Geometry check sheet. Reference: the model listing, model coordinates, mm. A direction names the side the tool comes from. Give positions to 0.01 mm unless a question says otherwise; leave off trailing zeros. Loops run counter-clockwise (first coordinate to the right, second up) from the corner with the lowest first, then second, coordinate; pieces in that order, holes last. Notation, with made-up numbers: (-17, 16.25) -> (2, 16.25) arc R4 ccw to (2, 20.25) -> close; hole circle Ø8 at (0.5, 35.25). An arc over 180 degrees is marked (long way). One line per item, written item: value. Start each with the question number.
(1) Sectioned sample at C-C, the plane y = 5.75. Record the cut outline in (x, z), then the cut area to 3 significant figures.
(2) Sectioned sample at D-D, the plane z = 0. State how many separate pieces and enclosed holes the cut face has, then the cut area to 3 significant figures.
(3) Gauge pin test, flat ends, axial feed: pin 1 Ø0.9 at (x, y) = (-4.5, -4) entering from +Z; pin 2 Ø1 at (y, z) = (-4.5, 0) entering from -X; pin 3 Ø4 at (x, z) = (-7.5, 2) entering from -Y (3 decimals). Record the tip position at first contact, or that the pin passes through.
(4) Sectioned sample at A-A, the plane x = -1.75. Record the cut outline in (y, z) (3 decimals), then the cut area to 3 significant figures.
(5) Draft check along Z on faces 1 (the face through (-4.544, -6.675, -0.011)), 2 (the face through (4.25, -5.3, -0.7)), 3 (the face through (0, 0, -3.4)). Enter one of: pulls with the +Z half, pulls with the -Z half, needs draft (parallel to the pull), parting line crosses it, or undercut.
(6) Tool access check on faces 4 (the face through (-4.544, -4.675, 0.011)), 5 (the face through (-7, 3.025, 0)), 6 (the face through (-0.35, -5.3, -0.7)), 7 (the face through (3.1, 6, 0)). Record the directions out of +Z, -Z, +X, -X, +Y, -Y that give a thin tool (end or side, any length) a straight path to the whole face; none if there is none.
(7) Sectioned sample at B-B, the plane z = -2.5. Record the cut outline in (x, y) (3 decimals), then the cut area to 3 significant figures.
(8) Scan lines: line 1 along X through (y, z) = (-4, -0.5); line 2 along Y through (x, z) = (5, 0) (3 decimals). Record each from-to range of solid material in increasing order. Write a range as from..to.
from build123d import *

# Parameters (mm, degrees)
BOSS_EXTRU_1_DEPTH      = 3.4
BOSS_EXTRU_1_DEPTH_BACK = 3.4
ENL_V_MAT_EXTRU_1_DEPTH = 6.8
ESQUISSE4_W             = 6.2
ESQUISSE4_H             = 4.2
ENL_V_MAT_EXTRU_2_DEPTH = 0.3
BOSS_EXTRU_2_DEPTH      = 1.95
BOSS_EXTRU_2_DEPTH_BACK = 1.95
ESQUISSE7_W             = 0.8
ESQUISSE7_H             = 2
BOSS_EXTRU_3_DEPTH      = 4.2
CONG_1_R                = 0.5
ENL_V_MAT_EXTRU_3_DEPTH = 10.2


with BuildPart() as part:
    # Esquisse1 → Boss.-Extru.1 (new body, two sides)
    with BuildSketch(Plane.XY) as boss_extru_1_sk:
        Polygon((-6.45, 3.275), (6.45, 3.275), (9.85, 3.275), (9.85, 3.025), (6.45, 3.025), (6.45, -3.275), (-6.45, -3.275), (-6.45, 3.025), (-9.85, 3.025), (-9.85, 3.275), align=None)
    extrude(amount=BOSS_EXTRU_1_DEPTH)
    extrude(boss_extru_1_sk.sketch, amount=-BOSS_EXTRU_1_DEPTH_BACK)

    # Esquisse3 → Enl_v. mat.-Extru.1 (cut)
    with BuildSketch(Plane(origin=(0, 3.275, 0), x_dir=(1, 0, 0), z_dir=(0, 1, 0))):
        with BuildLine():
            Line((-9.05, 1.2), (-9.85, 1.2))
            Line((-9.85, 1.2), (-9.85, -1.2))
            Line((-9.85, -1.2), (-9.05, -1.2))
            ThreePointArc((-9.05, -1.2), (-7.85, 0), (-9.05, 1.2))
        make_face()
        with BuildLine():
            Line((9.05, -1.2), (9.85, -1.2))
            Line((9.85, -1.2), (9.85, 1.2))
            Line((9.85, 1.2), (9.05, 1.2))
            ThreePointArc((9.05, 1.2), (7.85, 0), (9.05, -1.2))
        make_face()
    extrude(amount=-ENL_V_MAT_EXTRU_1_DEPTH, mode=Mode.SUBTRACT)

    # Esquisse4 → Enl_v. mat.-Extru.2 (cut)
    with BuildSketch(Plane(origin=(0, 3.275, 0), x_dir=(1, 0, 0), z_dir=(0, 1, 0))):
        Rectangle(ESQUISSE4_W, ESQUISSE4_H)
    extrude(amount=-ENL_V_MAT_EXTRU_2_DEPTH, mode=Mode.SUBTRACT)

    # Esquisse6 → Boss.-Extru.2 (add, two sides)
    with BuildSketch(Plane.XY) as boss_extru_2_sk:
        with BuildLine():
            Line((-0.8, 2.975), (3.1, 2.975))
            Line((3.1, 2.975), (3.1, 8.275))
            ThreePointArc((3.1, 8.275), (3.084706872, 8.281447306), (3.069392428, 8.287843813))
            Line((3.069392428, 8.287843813), (2.813852393, 8.173324546))
            Line((2.813852393, 8.173324546), (2.694192526, 8.426498179))
            ThreePointArc((2.694192526, 8.426498179), (2.674028844, 8.432998384), (2.6538378, 8.439413095))
            Line((2.6538378, 8.439413095), (2.409418963, 8.302757307))
            Line((2.409418963, 8.302757307), (2.267851834, 8.544364675))
            ThreePointArc((2.267851834, 8.544364675), (2.247192567, 8.549057375), (2.226513602, 8.553662498))
            Line((2.226513602, 8.553662498), (1.995128872, 8.395939706))
            Line((1.995128872, 8.395939706), (1.832762436, 8.624089904))
            ThreePointArc((1.832762436, 8.624089904), (1.811769271, 8.626938372), (1.790764225, 8.629697865))
            Line((1.790764225, 8.629697865), (1.574224502, 8.452142463))
            Line((1.574224502, 8.452142463), (1.392329497, 8.665049906))
            ThreePointArc((1.392329497, 8.665049906), (1.371166734, 8.66603185), (1.35, 8.666924116))
            Line((1.35, 8.666924116), (1.15, 8.470925717))
            Line((1.15, 8.470925717), (0.95, 8.666924116))
            ThreePointArc((0.95, 8.666924116), (0.928833266, 8.66603185), (0.907670503, 8.665049906))
            Line((0.907670503, 8.665049906), (0.725775498, 8.452142463))
            Line((0.725775498, 8.452142463), (0.509235775, 8.629697865))
            ThreePointArc((0.509235775, 8.629697865), (0.488230729, 8.626938372), (0.467237564, 8.624089904))
            Line((0.467237564, 8.624089904), (0.304871128, 8.395939706))
            Line((0.304871128, 8.395939706), (0.073486398, 8.553662498))
            ThreePointArc((0.073486398, 8.553662498), (0.052807433, 8.549057375), (0.032148166, 8.544364675))
            Line((0.032148166, 8.544364675), (-0.109418963, 8.302757307))
            Line((-0.109418963, 8.302757307), (-0.3538378, 8.439413095))
            ThreePointArc((-0.3538378, 8.439413095), (-0.374028844, 8.432998384), (-0.394192526, 8.426498179))
            Line((-0.394192526, 8.426498179), (-0.513852393, 8.173324546))
            Line((-0.513852393, 8.173324546), (-0.769392428, 8.287843813))
            ThreePointArc((-0.769392428, 8.287843813), (-0.784706872, 8.281447306), (-0.8, 8.275))
            Line((-0.8, 8.275), (-0.8, 2.975))
        make_face()
    extrude(amount=BOSS_EXTRU_2_DEPTH)
    extrude(boss_extru_2_sk.sketch, amount=-BOSS_EXTRU_2_DEPTH_BACK)

    # Esquisse7 → Boss.-Extru.3 (add)
    with BuildSketch(Plane.XZ.offset(3.275)):
        with Locations((-4.55, 0)):
            Rectangle(ESQUISSE7_W, ESQUISSE7_H)
        with Locations((0.05, 0)):
            Rectangle(ESQUISSE7_W, ESQUISSE7_H)
        with Locations((4.65, 0)):
            Rectangle(ESQUISSE7_W, ESQUISSE7_H)
    extrude(amount=BOSS_EXTRU_3_DEPTH)

    # Cong_1
    cong_1_edges = [part.edges().sort_by_distance(p)[0] for p in [
        (-4.55, -7.475, -1),
        (-4.55, -7.475, 1),
        (0.05, -7.475, 1),
        (0.05, -7.475, -1),
        (4.65, -7.475, 1),
        (4.65, -7.475, -1),
    ]]
    fillet(cong_1_edges, radius=CONG_1_R)

    # Esquisse8 → Enl_v. mat.-Extru.3 (cut)
    with BuildSketch(Plane(origin=(5.05, 0, 0), x_dir=(0, 0, -1), z_dir=(1, 0, 0))):
        with BuildLine():
            Line((0.5, -5.175), (0.5, -6.175))
            ThreePointArc((0.5, -6.175), (0, -6.675), (-0.5, -6.175))
            Line((-0.5, -6.175), (-0.5, -5.175))
            ThreePointArc((-0.5, -5.175), (0, -4.675), (0.5, -5.175))
        make_face()
    extrude(amount=-ENL_V_MAT_EXTRU_3_DEPTH, mode=Mode.SUBTRACT)


solid = part.part
Calculated:
1. outline: (-0.8, -1.95) -> (3.1, -1.95) -> (3.1, 1.95) -> (-0.8, 1.95) -> close
1. area: 15.2 mm2
2. separate pieces: 4
2. enclosed holes: 0
2. area: 110 mm2
3. pin 1: stops at z = 1
3. pin 2: stops at x = -4.95
3. pin 3: stops at y = -3.275
4. outline: (-3.275, -3.4) -> (3.275, -3.4) -> (3.275, -2.1) -> (2.975, -2.1) -> (2.975, 2.1) -> (3.275, 2.1) -> (3.275, 3.4) -> (-3.275, 3.4) -> close
4. area: 43.3 mm2
5. face 1: undercut
5. face 2: needs draft
5. face 3: pulls with the -Z half
6. face 4: +X, -X
6. face 5: +Z, -Z, -X, -Y
6. face 6: +Z, -Z, -Y
6. face 7: +Z, -Z, +X, +Y
7. outline: (-9.85, 3.025) -> (-6.45, 3.025) -> (-6.45, -3.275) -> (6.45, -3.275) -> (6.45, 3.025) -> (9.85, 3.025) -> (9.85, 3.275) -> (-9.85, 3.275) -> close
7. area: 86.2 mm2
8. line 1: x = -4.95..-4.15, -0.35..0.45, 4.25..5.05
8. line 2: y = -7.475..-6.675, -4.675..3.275
